Input: dimensioned drawing with shaded views. Units: mm. Origin: part minimum x, y, z. A direction names the side the tool comes from. Coordinates: 2 decimals unless noted, no trailing zeros. Write each loop counter-clockwise with the first axis right and the second up, starting at its lowest first coordinate (ties: lowest second). Pieces come first, ordered by that corner, then holes. Notation, with made-up numbers: (-13.75, 43.25) -> (22.25, 43.25) arc R25 cw to (22.25, 75.25) -> close; hole circle Ø9 at (-1.75, -21.5). An arc over 180 degrees is marked (long way). One line per item, written item: value. Start each with the question number.
1. First-contact query: P1, Ø12, axis at y = 11.5, z = 23, coming from the -X side; P2, Ø11, axis at y = 3.5, z = 12, coming from the -X side; P3, Ø1.6, axis at x = 68, y = 17, coming from the -Z side. Flat tips, straight axial feed; report the tip coordinate or a pass-through.
2. Mould query, pull axis X, two halves, no side actions, for the marked faces 3, 4, 5 and 6. Classes: released by +X, released by -X, zero draft, split by the parting line, or undercut.
3. Section query C-C, the plane x = 35.5. Output: boundary loops of the cut face in (y, z).
4. Section query B-B, the plane y = 14. Output: boundary loops of the cut face in (x, z).
5. Section query D-D, the plane y = 8. Output: boundary loops of the cut face in (x, z), and give its area (3 significant figures).
6. Access query for the marked faces 1 and 2. Directions: +Z, -Z, +X, -X, +Y, -Y. A direction counts if a zero-diameter tool reaches every point of the face in a straight line with its end or side. Return the directions, or none.
7. Section query A-A, the plane z = 35.5. Output: boundary loops of the cut face in (x, y), and give its area (3 significant figures).
8. Line query: line 1 (Y direction, x = 0.9, z = 35.5); line 2 (Y direction, x = 22, z = 31.5); line 3 (Y direction, x = 25.5, z = 6). Output: solid intervals per line, ascending.
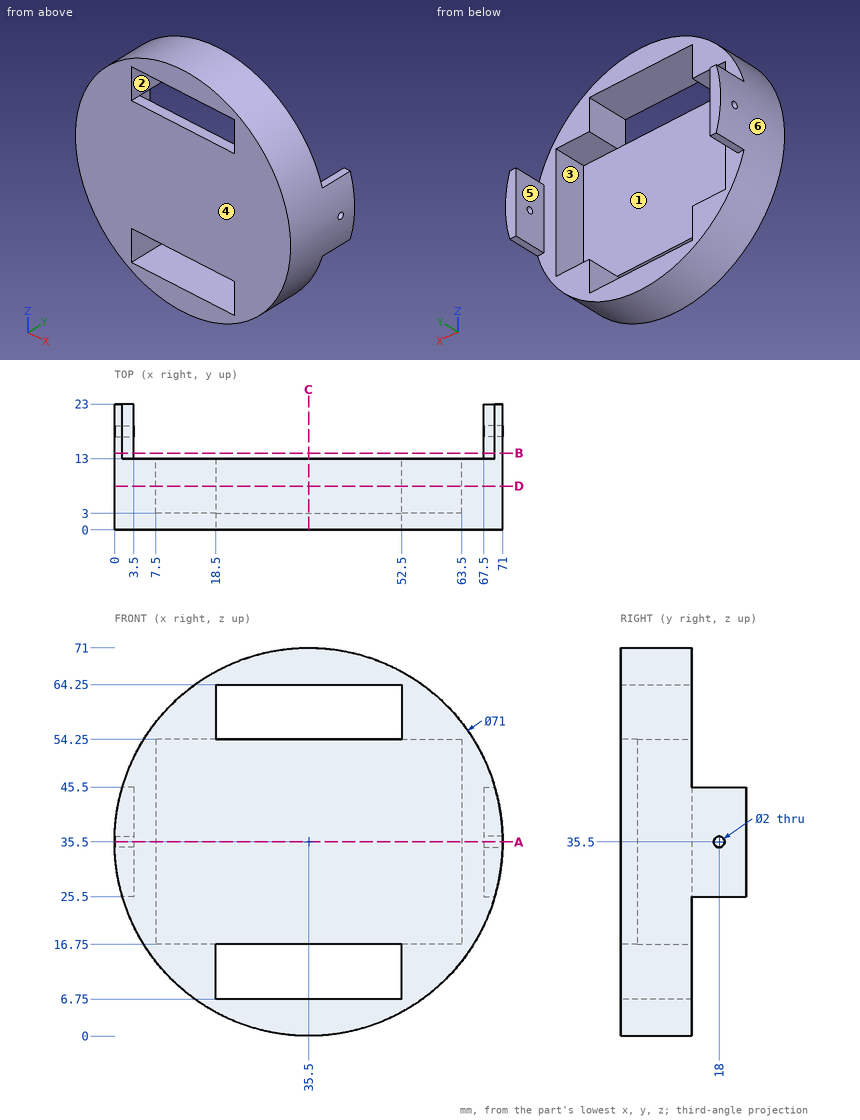
Computed values:
1. P1: stops at x = 0.6
1. P2: stops at x = 4.9
1. P3: stops at z = 25.5
2. face 3: undercut
2. face 4: zero draft
2. face 5: undercut
2. face 6: split by the parting line
3. outline: (0, 0) -> (13, 0) -> (13, 6.75) -> (0, 6.75) -> close; (0, 16.75) -> (3, 16.75) -> (3, 54.25) -> (0, 54.25) -> close; (0, 64.25) -> (13, 64.25) -> (13, 71) -> (0, 71) -> close
4. outline: (1.44, 25.5) -> (3.5, 25.5) -> (3.5, 45.5) -> (1.44, 45.5) arc R35.5 ccw to start; (67.5, 25.5) -> (69.56, 25.5) arc R35.5 ccw to (69.56, 45.5) -> (67.5, 45.5) -> close
5. outline: circle Ø71 at (35.5, 35.5); hole (7.5, 16.75) -> (18.5, 16.75) -> (18.5, 6.75) -> (52.5, 6.75) -> (52.5, 16.75) -> (63.5, 16.75) -> (63.5, 54.25) -> (52.5, 54.25) -> (52.5, 64.25) -> (18.5, 64.25) -> (18.5, 54.25) -> (7.5, 54.25) -> close
5. area: 1,180 mm²
6. face 1: +Y
6. face 2: +Y, -Y
7. outline: (0, 0) -> (71, 0) -> (71, 17) -> (67.5, 17) -> (67.5, 13) -> (63.5, 13) -> (63.5, 3) -> (7.5, 3) -> (7.5, 13) -> (3.5, 13) -> (3.5, 17) -> (0, 17) -> close; (0, 19) -> (3.5, 19) -> (3.5, 23) -> (0, 23) -> close; (67.5, 19) -> (71, 19) -> (71, 23) -> (67.5, 23) -> close
7. area: 419 mm²
8. line 1: y = 0 to 17, 19 to 23
8. line 2: y = 0 to 3
8. line 3: y = 0 to 13
